from build123d import *

# Parameters (mm, degrees)
F0_W      = 94.72
F0_H      = 45
F1_DEPTH  = 1.5
F3_D      = 3.935
F3_DEPTH  = 25.4
F3_TIP    = 1.1821932679
F4_D      = 3.935
F4_DEPTH  = 25.4
F4_TIP    = 1.1821932679
F5_W      = 50
F5_H      = 12.7415785939
F6_DEPTH  = 25.4
F7_R      = 5.08
F8_W      = 50
F8_H      = 15.24
F9_DEPTH  = 25.4
F10_W     = 11.9
F10_H     = 5
F11_DEPTH = 25.4
F12_W     = 3.81
F12_H     = 5.5
F13_DEPTH = 23
F14_W     = 4.5235089016
F14_H     = 3.4214928448
F15_DEPTH = 22.86
F16_W     = 4.5235114
F16_H     = 3.429
F17_DEPTH = 22.86
F18_W     = 2.0578785336
F18_H     = 3.2914727926
F19_DEPTH = 0.762
F20_W     = 49.26
F20_H     = 1.5
F21_DEPTH = 22.9616
F22_W     = 4
F22_H     = 1.0637021292
F23_DEPTH = 2.54
F24_W     = 1.9
F24_H     = 27.3218312255
F25_DEPTH = 25.4
F26_W     = 1.905
F26_H     = 20.46
F27_DEPTH = 1.651
F28_W     = 1.905
F28_H     = 20.46
F29_DEPTH = 3.048


with BuildPart() as f1:
    # F0 (on Top) → F1 (new body)
    with BuildSketch(Plane.XY):
        Rectangle(F0_W, F0_H)
    extrude(amount=F1_DEPTH)

    # F3
    with Locations(Plane.XY.offset(1.5)):
        with Locations((-31.3515785038, 8.1213163212)):
            Hole(F3_D / 2, depth=F3_DEPTH)
            with Locations((0, 0, -(F3_DEPTH + F3_TIP / 2))):  # 118° drill point
                Cone(0, F3_D / 2, F3_TIP, mode=Mode.SUBTRACT)

    # F4
    with Locations(Plane.XY.offset(1.5)):
        with Locations((30.1484214962, 8.1213163212)):
            Hole(F4_D / 2, depth=F4_DEPTH)
            with Locations((0, 0, -(F4_DEPTH + F4_TIP / 2))):  # 118° drill point
                Cone(0, F4_D / 2, F4_TIP, mode=Mode.SUBTRACT)

    # F5 (on face) → F6 (cut)
    with BuildSketch(Plane.XY.offset(1.5)):
        with Locations((0, 16.1292107031)):
            Rectangle(F5_W, F5_H)
    extrude(amount=-F6_DEPTH, mode=Mode.SUBTRACT)

    # F7
    f7_edges = [f1.edges().sort_by_distance(p)[0] for p in [
        (-47.36, -22.5, 0.75),
        (47.36, -22.5, 0.75),
    ]]
    fillet(f7_edges, radius=F7_R)

    # F8 (on face) → F9 (cut)
    with BuildSketch(Plane.XY.offset(1.5)):
        with Locations((0, 2.7981687745)):
            Rectangle(F8_W, F8_H)
    extrude(amount=-F9_DEPTH, mode=Mode.SUBTRACT)

    # F10 (on face) → F11 (cut)
    with BuildSketch(Plane.XY.offset(1.5)):
        with Locations((0, -12.2533300715)):
            Rectangle(F10_W, F10_H)
    extrude(amount=-F11_DEPTH, mode=Mode.SUBTRACT)

    # F12 (on face) → F13 (join)
    with BuildSketch(Plane.XY.offset(1.5)):
        with Locations((-21.6960607332, -12.3569313288)):
            Rectangle(F12_W, F12_H)
        with Locations((23.7539392668, -12.3569313288)):
            Rectangle(F12_W, F12_H)
    extrude(amount=F13_DEPTH)

    # F14 (on face) → F15 (cut)
    with BuildSketch(Plane.XY.offset(24.5)):
        with Locations((-19.7910607332, -12.3569313288)):
            Rectangle(F14_W, F14_H)
    extrude(amount=-F15_DEPTH, mode=Mode.SUBTRACT)

    # F16 (on face) → F17 (cut)
    with BuildSketch(Plane.XY.offset(24.5)):
        with Locations((21.8489392668, -12.3569313288)):
            Rectangle(F16_W, F16_H)
    extrude(amount=-F17_DEPTH, mode=Mode.SUBTRACT)

    # F18 (on face) → F19 (cut)
    with BuildSketch(Plane.XY.offset(1.5)):
        Polygon((-19.7910607332, -10.7469186187), (-19.7910607332, -14.0432291996), (19.7910607332, -14.0432291996), (19.7910607332, -14.0383914113), (19.7910607332, -10.7469186187), align=None)
        with Locations((20.82, -12.392655015)):
            Rectangle(F18_W, F18_H)
    extrude(amount=-F19_DEPTH, mode=Mode.SUBTRACT)

    # F20 (on face) → F21 (join)
    with BuildSketch(Plane.XY.offset(1.5)):
        with Locations((1.0289392668, -8.8569313288)):
            Rectangle(F20_W, F20_H)
    extrude(amount=F21_DEPTH)

    # F22 (on face) → F23 (join)
    with BuildSketch(Plane.XY.offset(1.5)):
        with Locations((-17.7910607332, -14.5750802642)):
            Rectangle(F22_W, F22_H)
        with Locations((19.8489392668, -14.5750802642)):
            Rectangle(F22_W, F22_H)
    extrude(amount=F23_DEPTH)

    # F24 (on face) → F25 (cut)
    with BuildSketch(Plane.XY.offset(1.5)):
        with Locations((-25.95, 8.8390843872)):
            Rectangle(F24_W, F24_H)
        with Locations((25.95, 8.8390843872)):
            Rectangle(F24_W, F24_H)
    extrude(amount=-F25_DEPTH, mode=Mode.SUBTRACT)

    # F26 (on face) → F27 (cut)
    with BuildSketch(Plane.XZ.offset(15.1069313288)):
        with Locations((-20.7435607332, 14.27)):
            Rectangle(F26_W, F26_H)
    extrude(amount=-F27_DEPTH, mode=Mode.SUBTRACT)

    # F28 (on face) → F29 (cut)
    with BuildSketch(Plane.XZ.offset(15.1069313288)):
        with Locations((22.8014392668, 14.27)):
            Rectangle(F28_W, F28_H)
    extrude(amount=-F29_DEPTH, mode=Mode.SUBTRACT)


solid = f1.part
CAD build for the part. Positions are in the model's coordinates, mm. A direction names the side the tool comes from. Give positions to 0.01 mm unless a question says otherwise; leave off trailing zeros. Write each loop counter-clockwise with the first axis right and the second up, starting at its lowest first coordinate (ties: lowest second). Pieces come first, ordered by that corner, then holes. Notation, with made-up numbers: (-15, -20.75) - (36, -20.75) arc R21 ccw to (36, -14.75) - close; hole circle Ø5 at (57, -0.75). An arc over 180 degrees is marked (long way). Answer as CSV lines item,"result".
Q1. Band-saw the part on C-C (x = -30.5). Give the cut face in (y, z).
Result set:
outline,"(-22.5, 0) - (6.35, 0) - (6.35, 1.5) - (-22.5, 1.5) - close; (9.89, 0) - (22.5, 0) - (22.5, 1.5) - (9.89, 1.5) - close"
Q2. Drill centre lines: line 1 (X direction, y = -12, z = 5.75); line 2 (X direction, y = -14.5, z = 2); line 3 (Z direction, x = 13, y = -18). Where is each one in solid material? Low to high. Write a range as from..to.
Result set:
line 1,"-23.6..-22.05, 24.11..25.66"
line 2,"-23.6..-15.79, 17.85..25.66"
line 3,"0..1.5"
Q3. 3-axis set-ups, long thin cutter, end or side, ignore diameter. For faces 4 (the face through (-22, -15.107, 10)), 5 (the face through (25.659, -12, 13)), 6 (the face through (-21, -10.646, 13)), 7 (the face through (25, -12, 24.5)): which of +Z, -Z, +X, -X, +Y, -Y reach the whole face in a straight line?
Result set:
face 4,"+Z, +X, -X, -Y"
face 5,"+Z, +X, +Y, -Y"
face 6,"+Z"
face 7,"+Z, +X, -X, +Y, -Y"
Q4. Pull direction Y, two halves, no side cores. Call faces 1 (the face through (-22.053, -12, 13)), 2 (the face through (-23.601, -12, 13)), 3 (the face through (24, -15.107, 10)): released by +Y, released by -Y, zero draft, split by the parting line, or undercut.
Result set:
face 1,"undercut"
face 2,"zero draft"
face 3,"released by -Y"
Q5. Band-saw the part on B-B (z = 9). Give the cut face in (x, y), and give its area (3 significant figures).
Result set:
outline,"(-23.6, -15.11) - (-21.7, -15.11) - (-21.7, -14.07) - (-22.05, -14.07) - (-22.05, -10.65) - (-19.79, -10.65) - (-19.79, -9.61) - (21.85, -9.61) - (21.85, -10.64) - (24.11, -10.64) - (24.11, -14.07) - (23.75, -14.07) - (23.75, -15.11) - (25.66, -15.11) - (25.66, -8.11) - (-23.6, -8.11) - close"
area,"96.4 mm²"
Q6. Band-saw the part on A-A (y = 4). Give the cut face in (x, z), and give its area (3 significant figures).
Result set:
outline,"(-47.36, 0) - (-26.9, 0) - (-26.9, 1.5) - (-47.36, 1.5) - close; (26.9, 0) - (47.36, 0) - (47.36, 1.5) - (26.9, 1.5) - close"
area,"61.4 mm²"
Q7. Flat gauge pins, fed straight in: pin 1 Ø1.6 at (x, y) = (12.5, -8.5) entering from +Z; pin 2 Ø7 at (x, z) = (1, 14.5) entering from -Y; pin 3 Ø5.5 at (y, z) = (-13, 12.5) entering from +X. Where does each tip first touch, or does it go through?
Result set:
pin 1,"z = 24.46"
pin 2,"y = -9.61"
pin 3,"x = 25.66"
Q8. Band-saw the part on D-D (y = -13). Give the cut face in (x, z).
Result set:
outline,"(-47.36, 0) - (-5.95, 0) - (-5.95, 0.74) - (-19.79, 0.74) - (-19.79, 1.64) - (-22.05, 1.64) - (-22.05, 24.5) - (-23.6, 24.5) - (-23.6, 1.5) - (-47.36, 1.5) - close; (5.95, 0) - (47.36, 0) - (47.36, 1.5) - (25.66, 1.5) - (25.66, 24.5) - (24.11, 24.5) - (24.11, 1.64) - (21.85, 1.64) - (21.85, 0.74) - (5.95, 0.74) - close"
